Geometry check sheet. Reference: the model listing, model coordinates, mm. Face numbers are marked on the shaded views. A direction names the side the tool comes from. Give positions to 0.01 mm unless a question says otherwise; leave off trailing zeros. Write each loop counter-clockwise with the first axis right and the second up, starting at its lowest first coordinate (ties: lowest second). Pieces come first, ordered by that corner, then holes. Notation, with made-up numbers: M -18.5,68.25 L -5.5,68.25 A15 ccw -5.5,83.25 Z; hole C -6,4 d3. An arc over 180 degrees is marked long. One line per item, written item: value. Start each with the question number.
1. Cross-section at B-B on y = -61.5. Record the cut outline in (x, z).
2. Scan lines: line 1 (Y direction, x = 6.75, z = 9.5); line 2 (X direction, y = -21.5, z = -10.75); line 3 (Z direction, x = -0.25, y = -23.5). Record each from-to range of solid material in increasing order.
3. Gauge pin test, flat ends, axial feed: pin 1 (1.5 mm diameter, centred on x = 9, y = -25, fed in from -Z); pin 2 (2 mm diameter, centred on y = -14.5, z = -11.5, fed in from -X); pin 3 (1 mm diameter, centred on x = 10, y = -11, fed in from +Z); pin 4 (5 mm diameter, centred on x = -5.5, z = -10, fed in from -Y). Record the tip position at first contact, or that the pin passes through.
4. Tool access check on the marked faces 1, 2 and 3. Record the directions out of +Z, -Z, +X, -X, +Y, -Y that give a thin tool (end or side, any length) a straight path to the whole face; none if there is none.
5. Cross-section at C-C on y = 4.5. Record the cut outline in (x, z), then the cut area to 3 significant figures.
6. Cross-section at A-A on y = -44.5. Record the cut outline in (x, z).
from build123d import *

# Parameters (mm, degrees)
F0_R      = 12.45
F1_DEPTH  = 12
F2_R      = 14.5
F3_DEPTH  = 3
F4_R      = 9.95
F5_DEPTH  = 70
F7_DEPTH  = 20
F10_DEPTH = 23.8
F11_R     = 0.5


with BuildPart() as f1:
    # F0 (on Front) → F1 (new body)
    with BuildSketch(Plane.XZ):
        Circle(F0_R)
    extrude(amount=-F1_DEPTH)

    # F2 (on Front) → F3 (join)
    with BuildSketch(Plane.XZ):
        Circle(F2_R)
    extrude(amount=F3_DEPTH)

    # F4 (on face) → F5 (join)
    with BuildSketch(Plane.XZ.offset(3)):
        Circle(F4_R)
    extrude(amount=F5_DEPTH)

    # F6 (on face) → F7 (join)
    with BuildSketch(Plane.XZ.offset(3)):
        with BuildLine():
            Line((2, 9.7469225913), (2, 12.3389626793))
            ThreePointArc((2, 12.3389626793), (0, 12.5), (-2, 12.3389626793))
            Line((-2, 12.3389626793), (-2, 9.7469225913))
            ThreePointArc((-2, 9.7469225913), (0, 9.95), (2, 9.7469225913))
        make_face()
        with BuildLine():
            ThreePointArc((-7.3471313431, 6.7098555146), (-5.8484632603, 8.049719094), (-4.1110633656, 9.0609965238))
            Line((-4.1110633656, 9.0609965238), (-5.6346263027, 11.1580010051))
            ThreePointArc((-5.6346263027, 11.1580010051), (-7.3473156537, 10.1127124297), (-8.8706942802, 8.8068599959))
            Line((-8.8706942802, 8.8068599959), (-7.3471313431, 6.7098555146))
        make_face()
        with BuildLine():
            ThreePointArc((-9.887908233, 1.109851691), (-9.4630123371, 3.074719094), (-8.6518402555, 4.9140777561))
            Line((-8.6518402555, 4.9140777561), (-11.1170168717, 5.7150621934))
            ThreePointArc((-11.1170168717, 5.7150621934), (-11.8882064537, 3.8627124297), (-12.3530848492, 1.9108361283))
            Line((-12.3530848492, 1.9108361283), (-9.887908233, 1.109851691))
        make_face()
        with BuildLine():
            ThreePointArc((-8.6518402555, -4.9140777561), (-9.4630123371, -3.074719094), (-9.887908233, -1.109851691))
            Line((-9.887908233, -1.109851691), (-12.3530848492, -1.9108361283))
            ThreePointArc((-12.3530848492, -1.9108361283), (-11.8882064537, -3.8627124297), (-11.1170168717, -5.7150621934))
            Line((-11.1170168717, -5.7150621934), (-8.6518402555, -4.9140777561))
        make_face()
        with BuildLine():
            ThreePointArc((-4.1110633656, -9.0609965238), (-5.8484632603, -8.049719094), (-7.3471313431, -6.7098555146))
            Line((-7.3471313431, -6.7098555146), (-8.8706942802, -8.8068599959))
            ThreePointArc((-8.8706942802, -8.8068599959), (-7.3473156537, -10.1127124297), (-5.6346263027, -11.1580010051))
            Line((-5.6346263027, -11.1580010051), (-4.1110633656, -9.0609965238))
        make_face()
        with BuildLine():
            ThreePointArc((2, -9.7469225913), (0, -9.95), (-2, -9.7469225913))
            Line((-2, -9.7469225913), (-2, -12.3389626793))
            ThreePointArc((-2, -12.3389626793), (0, -12.5), (2, -12.3389626793))
            Line((2, -12.3389626793), (2, -9.7469225913))
        make_face()
        with BuildLine():
            Line((8.8706942802, -8.8068599959), (7.3471313431, -6.7098555146))
            ThreePointArc((7.3471313431, -6.7098555146), (5.8484632603, -8.049719094), (4.1110633656, -9.0609965238))
            Line((4.1110633656, -9.0609965238), (5.6346263027, -11.1580010051))
            ThreePointArc((5.6346263027, -11.1580010051), (7.3473156537, -10.1127124297), (8.8706942802, -8.8068599959))
        make_face()
        with BuildLine():
            Line((12.3530848492, -1.9108361283), (9.887908233, -1.109851691))
            ThreePointArc((9.887908233, -1.109851691), (9.4630123371, -3.074719094), (8.6518402555, -4.9140777561))
            Line((8.6518402555, -4.9140777561), (11.1170168717, -5.7150621934))
            ThreePointArc((11.1170168717, -5.7150621934), (11.8882064537, -3.8627124297), (12.3530848492, -1.9108361283))
        make_face()
        with BuildLine():
            Line((11.1170168717, 5.7150621934), (8.6518402555, 4.9140777561))
            ThreePointArc((8.6518402555, 4.9140777561), (9.4630123371, 3.074719094), (9.887908233, 1.109851691))
            Line((9.887908233, 1.109851691), (12.3530848492, 1.9108361283))
            ThreePointArc((12.3530848492, 1.9108361283), (11.8882064537, 3.8627124297), (11.1170168717, 5.7150621934))
        make_face()
        with BuildLine():
            Line((5.6346263027, 11.1580010051), (4.1110633656, 9.0609965238))
            ThreePointArc((4.1110633656, 9.0609965238), (5.8484632603, 8.049719094), (7.3471313431, 6.7098555146))
            Line((7.3471313431, 6.7098555146), (8.8706942802, 8.8068599959))
            ThreePointArc((8.8706942802, 8.8068599959), (7.3473156537, 10.1127124297), (5.6346263027, 11.1580010051))
        make_face()
    extrude(amount=F7_DEPTH)

    # F9 (on offset) → F10 (cut)
    with BuildSketch(Plane.XY.offset(6)):
        with BuildLine():
            Line((-3, -52.9026644758), (-3, -80.1426661679))
            Line((-3, -80.1426661679), (3, -80.1426661679))
            Line((3, -80.1426661679), (3, -52.9026644758))
            ThreePointArc((3, -52.9026644758), (0, -49.9026644758), (-3, -52.9026644758))
        make_face()
    extrude(amount=F10_DEPTH, mode=Mode.SUBTRACT)

    # F11
    f11_edges = [f1.edges().sort_by_distance(p)[0] for p in [
        (-3, -62.951332, 9.486965),
        (0, -49.902664, 9.95),
        (3, -62.951332, 9.486965),
        (-5.880157, -73, -8.026596),
    ]]
    fillet(f11_edges, radius=F11_R)


solid = f1.part
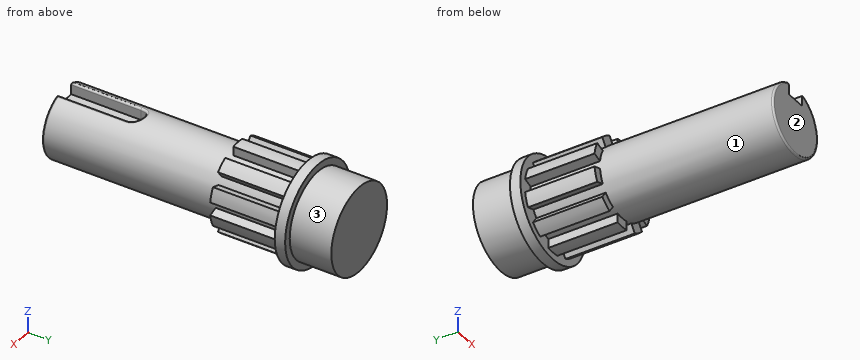
Report:
1. outline: M -3.69,9.24 A9.95 ccw long 3.69,9.24 A0.5 ccw 3,8.78 L 3,6 L -3,6 L -3,8.78 A0.5 ccw Z
2. line 1: y = -23 to 12
2. line 2: x = -6.38 to -5.34, -2 to 2, 5.34 to 6.38
2. line 3: z = -9.95 to 9.95
3. pin 1: stops at z = -5.56
3. pin 2: stops at x = -6.78
3. pin 3: stops at z = 5.51
3. pin 4: stops at y = -73
4. face 1: -Y
4. face 2: +Z, -Z, +X, -X, -Y
4. face 3: +Y
5. outline: C 0,0 d24.9
5. area: 487 mm^2
6. outline: C 0,0 d19.9
